Geometry: final body of the model. Coordinates: model frame, mm. A direction names the side the tool comes from. Round coordinates to 2 decimals unless told otherwise and drop trailing zeros. Loops run counter-clockwise (first coordinate to the right, second up) from the corner with the lowest first, then second, coordinate; pieces in that order, holes last. Notation, with made-up numbers: (5, 25) - (12, 25) arc R27 ccw to (12, 53) - close; hole circle Ø8 at (-7.75, 89.25). An arc over 180 degrees is marked (long way). Write item = value, one per line. Start each with the question number.
Item 1: Section C-C (x = 8.75). Return loops of the section in (y, z), plus the area to 3 significant figures.
Item 2: Draft query along Z for faces 4 (the flat face through (15, 28.272, -49)), 5 (the flat face through (2, 0, -21)), 6 (the flat face through (2, 3, 21.647)). Return one class per face: pulls with the +Z half, pulls with the -Z half, needs draft (parallel to the pull), parting line crosses it, or undercut.
Item 3: Access query for faces 1 (the flat face through (5, -3, -18)), 2 (the flat face through (12, 29, -36.762)), 3 (the flat face through (2, 3, -58.036)). Directions: +Z, -Z, +X, -X, +Y, -Y. A direction counts if a zero-diameter tool reaches every point of the face in a straight line with its end or side. Return the directions, or none.
Item 4: Section A-A (y = 9.5). Return loops of the section in (x, z).
Item 5: First-contact query: pin 1 (2.5 mm diameter, centred on x = 9.5, y = 29.5, fed in from +Z); pin 2 (5 mm diameter, centred on y = -13.5, z = -19.5, fed in from +X); pin 3 (4 mm diameter, centred on x = 6, y = 23.5, fed in from -Z). Flat tips, straight axial feed; report the tip coordinate or a pass-through.
Item 6: Line query: line 1 (Z direction, x = 2.75, y = 3.5); line 2 (X direction, y = -8, z = 15); line 3 (Z direction, x = 2.25, y = 24.5). Output: solid intervals per line, ascending. Write a range as from..to.
Item 7: Section B-B (z = -39.5). Return loops of the section in (x, y), plus the area to 3 significant figures.
Item 8: Section D-D (y = -3). Return loops of the section in (x, z), plus the area to 3 significant figures.
from build123d import *

# Parameters (mm, degrees)
F1_DEPTH = 5
F2_W     = 2.42595
F2_H     = 24.259482
F3_DEPTH = 25


with BuildPart() as f1:
    # F0 (on Right) → F1 (new body)
    with BuildSketch(Plane.YZ):
        Polygon((14.835605, 0), (14.648993, 21.646921), (-9.762866, 21.646921), (-21.926837, -6.904621), (-21.926837, -58.036141), (28.271621, -58.036141), (28.271621, -40.494673), (0, -40.494673), (0, 0), align=None)
    extrude(amount=F1_DEPTH)

    # F2 (on Right) → F3 (join)
    with BuildSketch(Plane.YZ):
        with Locations((29.484596, -48.892183)):
            Rectangle(F2_W, F2_H)
    extrude(amount=F3_DEPTH)


solid = f1.part
Taken from the geometry:
q1.outline = (28.27, -61.02) - (30.7, -61.02) - (30.7, -36.76) - (28.27, -36.76) - close
q1.area = 58.9 mm^2
q2.face_4 = needs draft
q2.face_5 = undercut
q2.face_6 = pulls with the +Z half
q3.face_1 = +Z, -Z, +X, -Y
q3.face_2 = +Z, +X, -X, +Y
q3.face_3 = -Z, +X, -X, -Y
q4.outline = (0, -58.04) - (5, -58.04) - (5, -40.49) - (0, -40.49) - close; (0, 0) - (5, 0) - (5, 21.65) - (0, 21.65) - close
q5.pin_1 = -36.76
q5.pin_2 = 5
q5.pin_3 = -58.04
q6.line_1 = -58.04..-40.49, 0..21.65
q6.line_2 = 0..5
q6.line_3 = -58.04..-40.49
q7.outline = (0, -21.93) - (5, -21.93) - (5, 0) - (0, 0) - close; (0, 28.27) - (25, 28.27) - (25, 30.7) - (0, 30.7) - close
q7.area = 170 mm^2
q8.outline = (0, -58.04) - (5, -58.04) - (5, 21.65) - (0, 21.65) - close
q8.area = 398 mm^2
